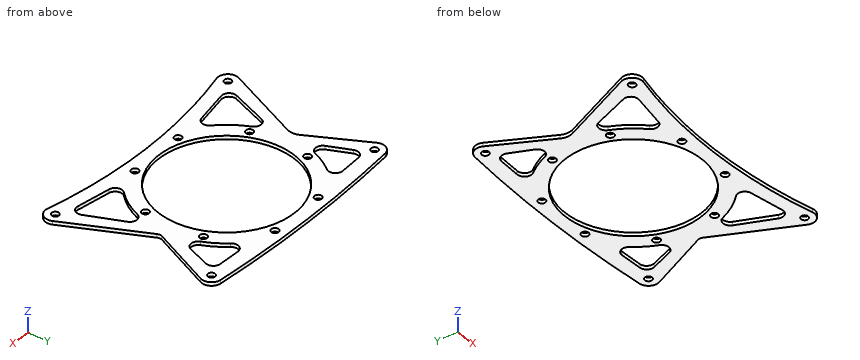
from build123d import *

# Parameters (mm, degrees)
SKETCH5_R           = 3.175
SKETCH5_R_2         = 3.25
SKETCH5_R_3         = 60.96
BOSS_EXTRUDE2_DEPTH = 3.175


with BuildPart() as part:
    # Sketch5 → Boss-Extrude2 (new body)
    with BuildSketch(Plane.XY):
        with BuildLine():
            Line((233.935091571, -114.763518579), (265.665701875, -184.883595476))
            ThreePointArc((265.665701875, -184.883595476), (264.423436425, -194.206670618), (255.505854783, -197.196602259))
            ThreePointArc((255.505854783, -197.196602259), (153.444246818, -185.249846144), (51.403286659, -197.37169633))
            ThreePointArc((51.403286659, -197.37169633), (42.43911219, -194.346602456), (41.276859828, -184.957417917))
            Line((41.276859828, -184.957417917), (72.669263517, -117.915407124))
            ThreePointArc((72.669263517, -117.915407124), (73.866746362, -112.37217505), (72.532031625, -106.860376473))
            Line((72.532031625, -106.860376473), (47.422094343, -56.527870305))
            ThreePointArc((47.422094343, -56.527870305), (47.614528636, -48.22631495), (54.579553655, -43.705111707))
            ThreePointArc((54.579553655, -43.705111707), (153.704366218, -39.249697911), (252.829178781, -43.705111707))
            ThreePointArc((252.829178781, -43.705111707), (259.764657482, -48.173800982), (260.039703094, -56.419672588))
            Line((260.039703094, -56.419672588), (233.987235662, -110.463230544))
            ThreePointArc((233.987235662, -110.463230544), (233.48365469, -112.607584422), (233.935091571, -114.763518579))
        make_face()
        with Locations((49.32793696, -188.727332639)):
            Circle(SKETCH5_R, mode=Mode.SUBTRACT)
        with Locations((55.377109151, -52.559263571)):
            Circle(SKETCH5_R, mode=Mode.SUBTRACT)
        with Locations((252.031623286, -52.559263571)):
            Circle(SKETCH5_R, mode=Mode.SUBTRACT)
        with Locations((90.880558007, -138.272171312)):
            Circle(SKETCH5_R_2, mode=Mode.SUBTRACT)
        with Locations((127.681892817, -175.073506122)):
            Circle(SKETCH5_R_2, mode=Mode.SUBTRACT)
        with Locations((179.726839619, -175.073506122)):
            Circle(SKETCH5_R_2, mode=Mode.SUBTRACT)
        with Locations((216.528174429, -138.272171312)):
            Circle(SKETCH5_R_2, mode=Mode.SUBTRACT)
        with Locations((216.528174429, -86.227224511)):
            Circle(SKETCH5_R_2, mode=Mode.SUBTRACT)
        with Locations((179.726839619, -49.425889701)):
            Circle(SKETCH5_R_2, mode=Mode.SUBTRACT)
        with Locations((127.681892817, -49.425889701)):
            Circle(SKETCH5_R_2, mode=Mode.SUBTRACT)
        with Locations((90.880558007, -86.227224511)):
            Circle(SKETCH5_R_2, mode=Mode.SUBTRACT)
        with Locations((153.704366218, -112.249697911)):
            Circle(SKETCH5_R_3, mode=Mode.SUBTRACT)
        with Locations((257.566369908, -188.548690521)):
            Circle(SKETCH5_R, mode=Mode.SUBTRACT)
        with BuildLine():
            Line((209.461649294, -176.161550354), (239.97260378, -181.443451933))
            ThreePointArc((239.97260378, -181.443451933), (245.991796239, -179.18128426), (246.949420177, -172.822743797))
            Line((246.949420177, -172.822743797), (234.263108846, -141.191675264))
            ThreePointArc((234.263108846, -141.191675264), (228.418953488, -137.205640522), (222.513375511, -141.100094727))
            ThreePointArc((222.513375511, -141.100094727), (215.504437403, -154.056113183), (206.086743584, -165.382660352))
            ThreePointArc((206.086743584, -165.382660352), (204.484912095, -171.801991039), (209.461649294, -176.161550354))
        make_face(mode=Mode.SUBTRACT)
        with BuildLine():
            Line((216.971221053, -55.043652894), (237.085867612, -55.91533392))
            ThreePointArc((237.085867612, -55.91533392), (242.165926056, -58.84665781), (242.677579376, -64.689419522))
            Line((242.677579376, -64.689419522), (234.586463913, -84.223100209))
            ThreePointArc((234.586463913, -84.223100209), (228.697518519, -88.14302122), (222.836263182, -84.181816295))
            ThreePointArc((222.836263182, -84.181816295), (217.987361181, -74.371977351), (211.755754133, -65.37687511))
            ThreePointArc((211.755754133, -65.37687511), (211.027446603, -58.526470596), (216.971221053, -55.043652894))
        make_face(mode=Mode.SUBTRACT)
        with BuildLine():
            Line((67.017865041, -181.584438257), (97.982666146, -176.188564905))
            ThreePointArc((97.982666146, -176.188564905), (102.953981644, -171.82534341), (101.348381832, -165.40866757))
            ThreePointArc((101.348381832, -165.40866757), (91.836215085, -153.955297436), (84.787438766, -140.841344712))
            ThreePointArc((84.787438766, -140.841344712), (78.896402882, -136.924728627), (73.037344469, -140.889021736))
            Line((73.037344469, -140.889021736), (60.042928393, -172.943053933))
            ThreePointArc((60.042928393, -172.943053933), (60.98652829, -179.31704224), (67.017865041, -181.584438257))
        make_face(mode=Mode.SUBTRACT)
        with BuildLine():
            Line((70.322864824, -55.91533392), (90.437511384, -55.043652894))
            ThreePointArc((90.437511384, -55.043652894), (96.381285834, -58.526470596), (95.652978303, -65.37687511))
            ThreePointArc((95.652978303, -65.37687511), (89.421371255, -74.371977351), (84.572469254, -84.181816295))
            ThreePointArc((84.572469254, -84.181816295), (78.711213917, -88.14302122), (72.822268524, -84.223100209))
            Line((72.822268524, -84.223100209), (64.73115306, -64.689419522))
            ThreePointArc((64.73115306, -64.689419522), (65.242806381, -58.84665781), (70.322864824, -55.91533392))
        make_face(mode=Mode.SUBTRACT)
    extrude(amount=BOSS_EXTRUDE2_DEPTH)


solid = part.part
Here's how the part is built. I have some questions about the finished solid (model axes, mm). Coordinates: 2 decimals unless noted, no trailing zeros. Order: outer loops, then holes, each group sorted by start corner. A loop starts at its lowest first (then second) coordinate and runs counter-clockwise, first axis right, second up.
Item 1: If we section it at D-D on z = 1.8: State how many separate pieces and enclosed holes the cut face has, plus the area to 3 significant figures.
Result sheet:
separate pieces: 1
enclosed holes: 17
area: 12,800 mm2
Item 2: If we section it at C-C on x = 149.5: List the corners of the cut face in (y, z) for me (3 decimals), plus the area to 3 significant figures.
Result sheet:
outline: (-185.271, 0) - (-173.065, 0) - (-173.065, 3.175) - (-185.271, 3.175) - close; (-51.435, 0) - (-39.258, 0) - (-39.258, 3.175) - (-51.435, 3.175) - close
area: 77.4 mm2
Item 3: If we section it at A-A on y = -147.5: List the corners of the cut face in (x, z) for me (3 decimals).
Result sheet:
outline: (58.816, 0) - (70.357, 0) - (70.357, 3.175) - (58.816, 3.175) - close; (87.944, 0) - (103.97, 0) - (103.97, 3.175) - (87.944, 3.175) - close; (203.439, 0) - (219.465, 0) - (219.465, 3.175) - (203.439, 3.175) - close; (236.793, 0) - (248.749, 0) - (248.749, 3.175) - (236.793, 3.175) - close
Item 4: I need wall thicknesses on line 1 (Y direction, x = 240.5, z = 0.65); line 2 (X direction, y = -144.5, z = 1.2); line 3 (Y direction, x = 232.5, z = 2.6). Which ranges of each line are inside material? Lowest first, please.
Result sheet:
line 1: y = -193.9 to -181.51, -156.74 to -129.27, -96.95 to -69.95, -57.09 to -42.66
line 2: x = 60.22 to 71.57, 86.42 to 101.97, 205.43 to 220.99, 235.59 to 247.39
line 3: y = -192.36 to -180.15, -138.73 to -86.9, -55.72 to -42.06
Item 5: If we section it at B-B on y = -122: List the corners of the cut face in (x, z) for me (3 decimals), plus the area to 3 significant figures.
Result sheet:
outline: (70.757, 0) - (93.529, 0) - (93.529, 3.175) - (70.757, 3.175) - close; (213.88, 0) - (237.21, 0) - (237.21, 3.175) - (213.88, 3.175) - close
area: 146 mm2
Item 6: For P1, Ø1.5, axis at x = 126, z = 2, coming from the -Y side, with a flat end and sliding along its axis, tell me the tip position at first contact or that it passes through.
Result sheet:
P1: stops at y = -186.18
